Geometry check sheet. Reference: the model listing, model coordinates, mm. A direction names the side the tool comes from. Round coordinates to 2 decimals unless told otherwise and drop trailing zeros. Order: outer loops, then holes, each group sorted by start corner. A loop starts at its lowest first (then second) coordinate and runs counter-clockwise, first axis right, second up.
(1) Cross-section at D-D on z = -0.45. Count the separate pieces of the cut face and the enclosed holes in it, and give its area (3 significant figures).
(2) Thickness scan on L1, parallel to Y at x = -5.5, z = -0.85; L2, parallel to X at y = -3.5, z = -1.65; L3, parallel to X at y = -2, z = -1.35. Record the ranges inside material, lowest first.
(3) Set-up check for faces 5 (the face through (-9, -3, 0)), 6 (the face through (-12.988, -3, -1)), 7 (the face through (-12.748, 2.384, -2.146)): record each of +Z, -Z, +X, -X, +Y, -Y from which the full face is reachable in a straight line by a thin tool's end or side.
(4) Cross-section at A-A on z = -3.7. Enter the section's corners in (x, y), and give its area (3 significant figures).
(5) Draft check along Y on faces 1 (the face through (-21, 3, 0)), 2 (the face through (11.51, -3.18, -2.54)), 3 (the face through (3.112, 0, -1)), 4 (the face through (-13.028, -2.366, -1.812)). Enter one of: pulls with the +Y half, pulls with the -Y half, needs draft (parallel to the pull), parting line crosses it, or undercut.
(6) Cross-section at B-B on y = 0. Enter the section's corners in (x, z), and give its area (3 significant figures).
(7) Cross-section at C-C on x = 2. Enter the section's corners in (y, z), and give its area (3 significant figures).
(8) Gauge pin test, flat ends, axial feed: P1, Ø0.6, axis at y = 3, z = -0.5, coming from the +X side; P2, Ø2.5, axis at y = 0, z = -1, coming from the -X side; P3, Ø1, axis at y = 3, z = -0.5, coming from the -X side. Record the tip position at first contact, or that the pin passes through.
from build123d import *

# Parameters (mm, degrees)
F0_W     = 1.5
F0_H     = 0.7
F0_R     = 2.25
F0_H_2   = 6.1
F0_W_2   = 2.8
F1_DEPTH = 5
F2_DEPTH = 3
F3_DEPTH = 2
F4_R     = 0.74999
F5_R     = 2


# Not quite as in the source:
# - a fillet or chamfer is up to 0.001 mm smaller than in the source, because OpenCascade refuses the exact size


with BuildPart() as f1:
    # F0 (on Top) → F1 (new body)
    with BuildSketch(Plane.XY):
        Polygon((-18.8879279066, 3.75), (-22.8879279066, 3.75), (-22.8879279066, 1.7), (-18.8879279066, 1.97), align=None)
        Polygon((-17.3879279066, 3.75), (-18.8879279066, 3.75), (-18.8879279066, 1.97), (-17.3879279066, 2.07125), align=None)
        Polygon((-18.8879279066, 1.97), (-22.8879279066, 1.7), (-22.8879279066, -1.7), (-18.8879279066, -1.97), align=None)
        Polygon((-12.9879279066, 3.75), (-17.3879279066, 3.75), (-17.3879279066, 2.07125), (-12.9879279066, 2.36825), align=None)
        Polygon((-18.8879279066, -1.97), (-22.8879279066, -1.7), (-22.8879279066, -3.75), (-18.8879279066, -3.75), align=None)
        Polygon((-11.4879279066, 3.75), (-12.9879279066, 3.75), (-12.9879279066, 2.36825), (-11.4879279066, 2.4695), align=None)
        Polygon((-17.3879279066, -2.07125), (-18.8879279066, -1.97), (-18.8879279066, -3.75), (-17.3879279066, -3.75), align=None)
        Polygon((-7.0879279066, 3.75), (-11.4879279066, 3.75), (-11.4879279066, 2.4695), (-7.0879279066, 2.7665), align=None)
        Polygon((-12.9879279066, -2.36825), (-17.3879279066, -2.07125), (-17.3879279066, -3.75), (-12.9879279066, -3.75), align=None)
        Polygon((-5.5879279066, 3.75), (-7.0879279066, 3.75), (-7.0879279066, 2.7665), (-5.5879279066, 2.86775), align=None)
        Polygon((-11.4879279066, -2.4695), (-12.9879279066, -2.36825), (-12.9879279066, -3.75), (-11.4879279066, -3.75), align=None)
        Polygon((-1.1879279066, 3.75), (-5.5879279066, 3.75), (-5.5879279066, 2.86775), (-2.8879279066, 3.05), (-1.1879279066, 3.05), align=None)
        Polygon((-7.0879279066, -2.7665), (-11.4879279066, -2.4695), (-11.4879279066, -3.75), (-7.0879279066, -3.75), align=None)
        with Locations((-0.4379279066, 3.4)):
            Rectangle(F0_W, F0_H)
        Polygon((-5.5879279066, -2.86775), (-7.0879279066, -2.7665), (-7.0879279066, -3.75), (-5.5879279066, -3.75), align=None)
        Polygon((12.1120720934, 3.75), (0.3120720934, 3.75), (0.3120720934, 3.05), (3.1120720934, 3.05), (3.1120720934, -3.05), (0.3120720934, -3.05), (0.3120720934, -3.75), (12.1120720934, -3.75), align=None)
        with Locations((8.1120720934, 0)):
            Circle(F0_R, mode=Mode.SUBTRACT)
        Polygon((-2.8879279066, -3.05), (-5.5879279066, -2.86775), (-5.5879279066, -3.75), (-1.1879279066, -3.75), (-1.1879279066, -3.05), align=None)
        with Locations((-0.4379279066, -3.4)):
            Rectangle(F0_W, F0_H)
        with Locations((-0.4379279066, 0)):
            Rectangle(F0_W, F0_H_2)
        Polygon((-5.5879279066, 2.86775), (-7.0879279066, 2.7665), (-7.0879279066, -2.7665), (-5.5879279066, -2.86775), align=None)
        Polygon((-17.3879279066, 2.07125), (-18.8879279066, 1.97), (-18.8879279066, -1.97), (-17.3879279066, -2.07125), align=None)
        Polygon((-12.9879279066, 2.36825), (-17.3879279066, 2.07125), (-17.3879279066, -2.07125), (-12.9879279066, -2.36825), align=None)
        Polygon((-7.0879279066, 2.7665), (-11.4879279066, 2.4695), (-11.4879279066, -2.4695), (-7.0879279066, -2.7665), align=None)
        Polygon((-11.4879279066, 2.4695), (-12.9879279066, 2.36825), (-12.9879279066, -2.36825), (-11.4879279066, -2.4695), align=None)
        Polygon((-2.8879279066, 3.05), (-5.5879279066, 2.86775), (-5.5879279066, -2.86775), (-2.8879279066, -3.05), (-1.1879279066, -3.05), (-1.1879279066, 3.05), align=None)
        with Locations((1.7120720934, 0)):
            Rectangle(F0_W_2, F0_H_2)
    extrude(amount=-F1_DEPTH)

    # F0 (on Top) → F2 (cut)
    with BuildSketch(Plane.XY):
        Polygon((-18.8879279066, 1.97), (-22.8879279066, 1.7), (-22.8879279066, -1.7), (-18.8879279066, -1.97), align=None)
        Polygon((-17.3879279066, 2.07125), (-18.8879279066, 1.97), (-18.8879279066, -1.97), (-17.3879279066, -2.07125), align=None)
        Polygon((-12.9879279066, 2.36825), (-17.3879279066, 2.07125), (-17.3879279066, -2.07125), (-12.9879279066, -2.36825), align=None)
        Polygon((-11.4879279066, 2.4695), (-12.9879279066, 2.36825), (-12.9879279066, -2.36825), (-11.4879279066, -2.4695), align=None)
        Polygon((-7.0879279066, 2.7665), (-11.4879279066, 2.4695), (-11.4879279066, -2.4695), (-7.0879279066, -2.7665), align=None)
        Polygon((-5.5879279066, 2.86775), (-7.0879279066, 2.7665), (-7.0879279066, -2.7665), (-5.5879279066, -2.86775), align=None)
        Polygon((-2.8879279066, 3.05), (-5.5879279066, 2.86775), (-5.5879279066, -2.86775), (-2.8879279066, -3.05), (-1.1879279066, -3.05), (-1.1879279066, 3.05), align=None)
        with Locations((-0.4379279066, 0)):
            Rectangle(F0_W, F0_H_2)
        with Locations((1.7120720934, 0)):
            Rectangle(F0_W_2, F0_H_2)
    extrude(amount=-F2_DEPTH, mode=Mode.SUBTRACT)

    # F0 (on Top) → F3 (cut)
    with BuildSketch(Plane.XY):
        Polygon((-17.3879279066, 3.75), (-18.8879279066, 3.75), (-18.8879279066, 1.97), (-17.3879279066, 2.07125), align=None)
        Polygon((-11.4879279066, 3.75), (-12.9879279066, 3.75), (-12.9879279066, 2.36825), (-11.4879279066, 2.4695), align=None)
        Polygon((-5.5879279066, 3.75), (-7.0879279066, 3.75), (-7.0879279066, 2.7665), (-5.5879279066, 2.86775), align=None)
        with Locations((-0.4379279066, -3.4)):
            Rectangle(F0_W, F0_H)
        Polygon((-17.3879279066, -2.07125), (-18.8879279066, -1.97), (-18.8879279066, -3.75), (-17.3879279066, -3.75), align=None)
        Polygon((-11.4879279066, -2.4695), (-12.9879279066, -2.36825), (-12.9879279066, -3.75), (-11.4879279066, -3.75), align=None)
        Polygon((-5.5879279066, -2.86775), (-7.0879279066, -2.7665), (-7.0879279066, -3.75), (-5.5879279066, -3.75), align=None)
        with Locations((-0.4379279066, 3.4)):
            Rectangle(F0_W, F0_H)
    extrude(amount=-F3_DEPTH, mode=Mode.SUBTRACT)

    # F4 (radius 0.75 in the source; OpenCascade refuses exactly that, so slightly less here)
    f4_edges = [f1.edges().sort_by_distance(p)[0] for p in [
        (-17.387928, -2.910625, -2),
        (-11.487928, -3.10975, -2),
        (-5.587928, -3.308875, -2),
        (0.312072, -3.4, -2),
        (-18.887928, -2.86, -2),
        (-12.987928, -3.059125, -2),
        (-7.087928, -3.25825, -2),
        (-1.187928, -3.4, -2),
        (-18.887928, 2.86, -2),
        (-12.987928, 3.059125, -2),
        (-7.087928, 3.25825, -2),
        (-1.187928, 3.4, -2),
        (-17.387928, 2.910625, -2),
        (-11.487928, 3.10975, -2),
        (-5.587928, 3.308875, -2),
        (0.312072, 3.4, -2),
        (3.112072, 3.05, -1.5),
        (3.112072, -3.05, -1.5),
    ]]
    fillet(f4_edges, radius=F4_R)

    # F5
    f5_edges = [f1.edges().sort_by_distance(p)[0] for p in [
        (-22.887928, -3.75, -2.5),
        (-22.887928, 3.75, -2.5),
        (12.112072, -3.75, -2.5),
        (12.112072, 3.75, -2.5),
    ]]
    fillet(f5_edges, radius=F5_R)


solid = f1.part
Found:
1. separate pieces: 9
1. enclosed holes: 1
1. area: 97.7 mm2
2. L1: y = -3.75 to -2.87, 2.87 to 3.75
2. L2: x = -21.86 to -18.77, -17.5 to -12.87, -11.6 to -6.97, -5.7 to -1.07, 0.2 to 11.08
2. L3: x = -22.87 to -18.88, 3.11 to 7.08, 9.14 to 12.1
3. face 5: +Z, +X, -X, +Y, -Y
3. face 6: +Z, +Y, -Y
3. face 7: +Z
4. outline: (-22.89, -1.75) arc R2 ccw to (-20.89, -3.75) - (10.11, -3.75) arc R2 ccw to (12.11, -1.75) - (12.11, 1.75) arc R2 ccw to (10.11, 3.75) - (-20.89, 3.75) arc R2 ccw to (-22.89, 1.75) - close; hole circle Ø4.5 at (8.11, 0)
4. area: 243 mm2
5. face 1: needs draft
5. face 2: pulls with the -Y half
5. face 3: undercut
5. face 4: undercut
6. outline: (-22.89, -5) - (5.86, -5) - (5.86, 0) - (3.11, 0) - (3.11, -3) - (-22.89, -3) - close; (10.36, -5) - (12.11, -5) - (12.11, 0) - (10.36, 0) - close
6. area: 74.5 mm2
7. outline: (-3.75, -5) - (3.75, -5) - (3.75, 0) - (3.05, 0) - (3.05, -3) - (-3.05, -3) - (-3.05, 0) - (-3.75, 0) - close
7. area: 19.2 mm2
8. P1: stops at x = 11.87
8. P2: stops at x = 3.11
8. P3: stops at x = -22.74
